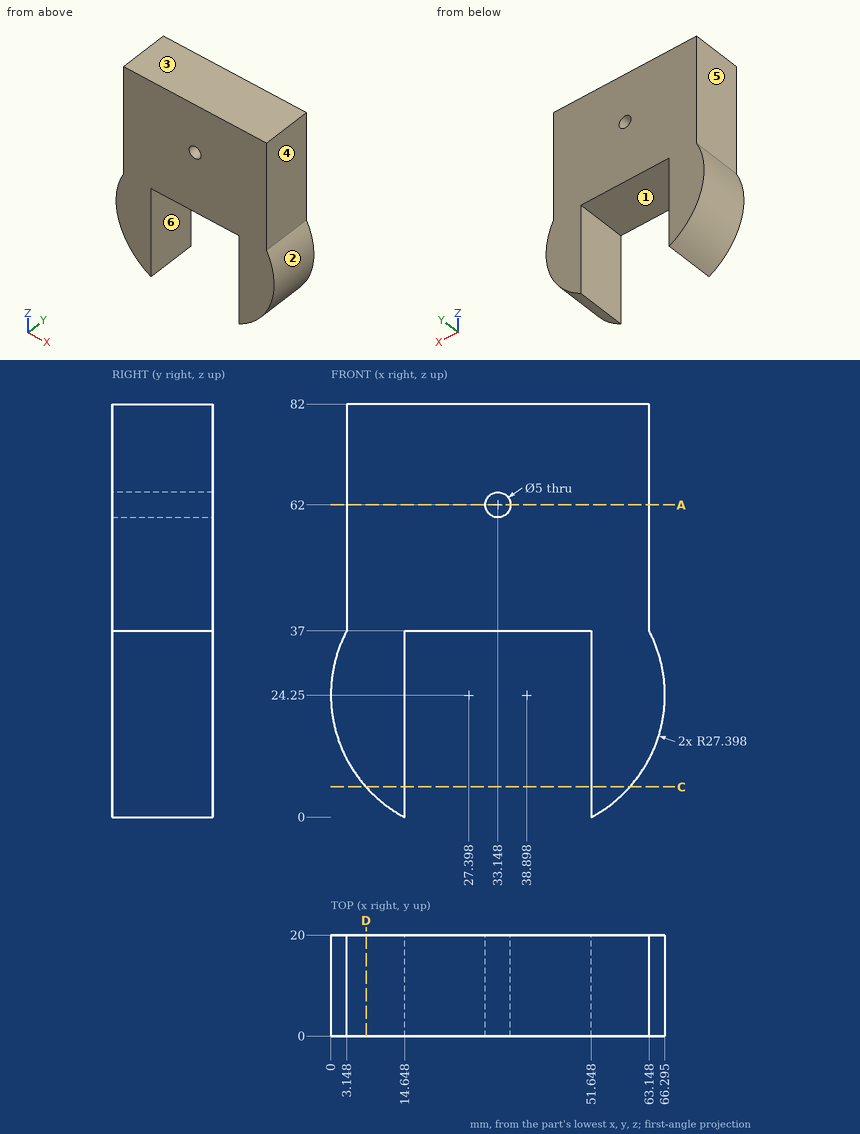
Job drawing, mm, ordinate dimensions from the low corner. One solid piece. A direction names the side the tool comes from. Round coordinates to 2 decimals unless told otherwise and drop trailing zeros. Loops run counter-clockwise (first coordinate to the right, second up) from the corner with the lowest first, then second, coordinate; pieces in that order, holes last. Notation, with made-up numbers: M 4.5,33 L 52.5,33 A14 ccw 52.5,38 Z; hole C -25,50 d9. An arc over 180 degrees is marked long. Answer as CSV lines item,"result".
1. Cut at C-C on z = 6. Write the cut outline in (x, y).
Resolved:
outline,"M 6.96,0 L 14.65,0 L 14.65,20 L 6.96,20 Z; M 51.65,0 L 59.33,0 L 59.33,20 L 51.65,20 Z"
2. Wall check: probe 1 along X at (y, z) = (10, 62); probe 2 along X at (y, z) = (2.5, 57.5); probe 3 along Z at (x, y) = (16.5, 12.5). Give the ranges that are in metal, low to high. Write a range as [from, to].
Resolved:
probe 1,"x = [3.15, 30.65], [35.65, 63.15]"
probe 2,"x = [3.15, 63.15]"
probe 3,"z = [37, 82]"
3. Cut at D-D on x = 7. Write the cut outline in (y, z).
Resolved:
outline,"M 0,5.96 L 20,5.96 L 20,82 L 0,82 Z"
4. Flat gauge pins, fed straight in: P1, Ø4, axis at y = 16.5, z = 13.5, coming from the +X side; P2, Ø10, axis at y = 17, z = 53, coming from the +X side; P3, Ø6, axis at y = 5.5, z = 55, coming from the -X side; P4, Ø12, axis at x = 19, z = 27.5, coming from the +Y side. Where does each tip first touch, or does it go through?
Resolved:
P1,"stops at x = 64.86"
P2,"stops at x = 63.15"
P3,"stops at x = 3.15"
P4,"stops at y = 20"
5. Two-plate mould, pull along X, no slides. Class the marked faces 3, 4, 5 and 6: released by +X, released by -X, zero draft, split by the parting line, or undercut.
Resolved:
face 3,"zero draft"
face 4,"released by +X"
face 5,"released by -X"
face 6,"undercut"
6. Cut at A-A on z = 62. Write the cut outline in (x, y), then the cut area to 3 significant figures.
Resolved:
outline,"M 3.15,0 L 30.65,0 L 30.65,20 L 3.15,20 Z; M 35.65,0 L 63.15,0 L 63.15,20 L 35.65,20 Z"
area,"1,100 mm²"
7. 3-axis set-ups, long thin cutter, end or side, ignore diameter. For the marked faces 1 and 2: which of +Z, -Z, +X, -X, +Y, -Y reach the whole face in a straight line?
Resolved:
face 1,"-Z, +Y, -Y"
face 2,"+X, +Y, -Y"
